```python
from build123d import *

# Parameters (mm, degrees)
F0_W     = 38
F0_H     = 16
F0_R     = 1.5
F1_DEPTH = 2
F2_SIZE  = 1.25
F4_R     = 5
F3_R     = 3
F3_R_2   = 1.5
F5_DEPTH = 1
F6_SIZE  = 0.5


with BuildPart() as f1:
    # F0 (on Top) → F1 (new body)
    with BuildSketch(Plane.XY):
        Rectangle(F0_W, F0_H)
        with Locations((-10, 0)):
            Circle(F0_R, mode=Mode.SUBTRACT)
        with Locations((10, 0)):
            Circle(F0_R, mode=Mode.SUBTRACT)
    extrude(amount=F1_DEPTH)

    # F2
    f2_edges = [f1.edges().sort_by_distance(p)[0] for p in [
        (0, -8, 2),
    ]]
    chamfer(f2_edges, length=F2_SIZE)

    # F4
    f4_edges = [f1.edges().sort_by_distance(p)[0] for p in [
        (19, 8, 1),
    ]]
    fillet(f4_edges, radius=F4_R)

    # F3 (on face) → F5 (cut)
    with BuildSketch(Plane.XY.offset(2)):
        with Locations((-10, 0)):
            Circle(F3_R)
        with Locations((-10, 0)):
            Circle(F3_R_2, mode=Mode.SUBTRACT)
    extrude(amount=-F5_DEPTH, mode=Mode.SUBTRACT)

    # F6
    f6_edges = [f1.edges().sort_by_distance(p)[0] for p in [
        (-2.5, 8, 0),
        (17.535534, 6.535534, 0),
        (-19, 0, 0),
        (19, -2.5, 0),
        (0, -8, 0),
        (-11.5, 0, 0),
        (8.5, 0, 0),
    ]]
    chamfer(f6_edges, length=F6_SIZE)


solid = f1.part
```
The model under review builds one solid part; all positions refer to its coordinate system, in mm. A direction names the side the tool comes from. Round coordinates to 2 decimals unless told otherwise and drop trailing zeros. Write each loop counter-clockwise with the first axis right and the second up, starting at its lowest first coordinate (ties: lowest second). Pieces come first, ordered by that corner, then holes. Notation, with made-up numbers: (64.5, 18) - (117.5, 18) arc R24 ccw to (117.5, 56) - close; hole circle Ø5 at (88, 40.25). An arc over 180 degrees is marked (long way). One line per question, with ' | ' between items.
Item 1: Add section B-B, the plane y = 0. Give the boundary of the cut face in (x, z), then the cut area to 4 significant figures.
Resolved:
outline: (-19, 0.5) - (-18.5, 0) - (-12, 0) - (-11.5, 0.5) - (-11.5, 1) - (-13, 1) - (-13, 2) - (-19, 2) - close; (-8.5, 0.5) - (-8, 0) - (8, 0) - (8.5, 0.5) - (8.5, 2) - (-7, 2) - (-7, 1) - (-8.5, 1) - close; (11.5, 0.5) - (12, 0) - (18.5, 0) - (19, 0.5) - (19, 2) - (11.5, 2) - close | area: 60.25 mm2
Item 2: For P1, Ø4, axis at x = -10, y = 0, coming from the +Z side; P2, Ø5, axis at x = 10, y = 0, coming from the -Z side, all flat-tipped, find the tip position at first contact; note any pin that passes through.
Resolved:
P1: stops at z = 1 | P2: stops at z = 0
Item 3: Add section C-C, the plane x = -14. Give the boundary of the cut face in (y, z), then the cut area to 3 significant figures.
Resolved:
outline: (-8, 0.5) - (-7.5, 0) - (7.5, 0) - (8, 0.5) - (8, 2) - (-6.75, 2) - (-8, 0.75) - close | area: 31.0 mm2
Item 4: Add section D-D, the plane x = 10. Give the boundary of the cut face in (y, z).
Resolved:
outline: (-8, 0.5) - (-7.5, 0) - (-2, 0) - (-1.5, 0.5) - (-1.5, 2) - (-6.75, 2) - (-8, 0.75) - close; (1.5, 0.5) - (2, 0) - (7.5, 0) - (8, 0.5) - (8, 2) - (1.5, 2) - close
Item 5: For faces 4 (the face through (-12.4, -1.8, 1.5)), 5 (the face through (17, 7, 1)), list the 3-axis set-ups (+Z, -Z, +X, -X, +Y, -Y) from which the entire face can be reached by the end or side of a thin tool; tool diameter is ignored.
Resolved:
face 4: +Z | face 5: +Z, -Z, +X, +Y
Item 6: To check wall thickness, follow probe 1 along Y at (x, z) = (10, 1.25); probe 2 along X at (y, z) = (-2.5, 1.75); probe 3 along X at (y, z) = (-0.25, 0.3). State the ranges of each line that lie inside material, in increasing order.
Resolved:
probe 1: y = -7.5 to -1.5, 1.5 to 8 | probe 2: x = -19 to -11.66, -8.34 to 19 | probe 3: x = -18.8 to -11.68, -8.32 to 8.32, 11.68 to 18.8
Item 7: Add section A-A, the plane x = -10. Give the boundary of the cut face in (y, z).
Resolved:
outline: (-8, 0.5) - (-7.5, 0) - (-2, 0) - (-1.5, 0.5) - (-1.5, 1) - (-3, 1) - (-3, 2) - (-6.75, 2) - (-8, 0.75) - close; (1.5, 0.5) - (2, 0) - (7.5, 0) - (8, 0.5) - (8, 2) - (3, 2) - (3, 1) - (1.5, 1) - close
Item 8: The part is to be moulded in two halves that separate along Y. For faces 1 (the face through (-19, 0, 1)), 2 (the face through (-8.7, -1.3, 1)), 3 (the face through (17.246, 6.319, 0.142)), say which applies: pulls with the +Y half, pulls with the -Y half, needs draft (parallel to the pull), parting line crosses it, or undercut.
Resolved:
face 1: needs draft | face 2: undercut | face 3: pulls with the +Y half
